from build123d import *

# Parameters (mm, degrees)
CROQUIS1_R                 = 15.5
CROQUIS1_R_2               = 1.5
SALIENTE_EXTRUIR1_DEPTH    = 18.25
CROQUIS2_R                 = 9
CORTAR_EXTRUIR1_DEPTH      = 10
CROQUIS3_R                 = 16.5
CROQUIS3_R_2               = 15.5
SALIENTE_EXTRUIR2_DEPTH    = 1.5
SALIENTE_EXTRUIR3_START    = -1.5
CROQUIS4_R                 = 16.5
CROQUIS4_R_2               = 15.5
SALIENTE_EXTRUIR3_DEPTH    = 1.5
CROQUIS5_W                 = 3
CROQUIS5_H                 = 6.34
CORTAR_EXTRUIR2_DEPTH      = 6.25
CORTAR_EXTRUIR3_DEPTH      = 8
CORTAR_EXTRUIR3_DEPTH_BACK = 9.75
CROQUIS7_R                 = 1.625
CROQUIS8_R                 = 1.625
CORTAR_EXTRUIR4_DEPTH      = 8.25
CORTAR_EXTRUIR7_START      = 15.25
CROQUIS9_R                 = 15.5
CROQUIS9_R_2               = 14.5
CORTAR_EXTRUIR7_DEPTH      = 15.25
CROQUIS11_R                = 16.5
CROQUIS11_R_2              = 9
SALIENTE_EXTRUIR4_DEPTH    = 3.75
CROQUIS12_R                = 16.5
CROQUIS12_R_2              = 14.5
CORTAR_EXTRUIR8_DEPTH      = 3.75


with BuildPart() as part:
    # Croquis1 → Saliente-Extruir1 (new body)
    with BuildSketch(Plane.XY):
        with Locations((-6.34746922, -2.918376653)):
            Circle(CROQUIS1_R)
        with Locations((-6.34746922, -2.918376653)):
            Circle(CROQUIS1_R_2, mode=Mode.SUBTRACT)
    extrude(amount=-SALIENTE_EXTRUIR1_DEPTH)

    # Croquis2 → Cortar-Extruir1 (cut)
    with BuildSketch(Plane(origin=(0, 0, -18.25), x_dir=(-1, 0, 0), z_dir=(0, 0, -1))):
        with Locations((6.34746922, -2.918376653)):
            Circle(CROQUIS2_R)
    extrude(amount=-CORTAR_EXTRUIR1_DEPTH, mode=Mode.SUBTRACT)

    # Croquis3 → Saliente-Extruir2 (add)
    with BuildSketch(Plane.XY):
        with Locations((-6.34746922, -2.918376653)):
            Circle(CROQUIS3_R)
        with Locations((-6.34746922, -2.918376653)):
            Circle(CROQUIS3_R_2, mode=Mode.SUBTRACT)
    extrude(amount=-SALIENTE_EXTRUIR2_DEPTH)

    # Croquis4 → Saliente-Extruir3 (add)
    with BuildSketch(Plane(origin=(0, 0, -18.25), x_dir=(-1, 0, 0), z_dir=(0, 0, -1)).offset(SALIENTE_EXTRUIR3_START)):
        with Locations(Location((6.34746922, -2.918376653, 0), (0, 0, 180))):
            Circle(CROQUIS4_R)
        with Locations(Location((6.34746922, -2.918376653, 0), (0, 0, 180))):
            Circle(CROQUIS4_R_2, mode=Mode.SUBTRACT)
    extrude(amount=SALIENTE_EXTRUIR3_DEPTH)

    # Croquis5 → Cortar-Extruir2 (cut)
    with BuildSketch(Plane.XY):
        with Locations((-0.34746922, -2.918376653)):
            Rectangle(CROQUIS5_W, CROQUIS5_H)
    extrude(amount=-CORTAR_EXTRUIR2_DEPTH, mode=Mode.SUBTRACT)

    # Croquis7 → Cortar-Extruir3 (cut, two sides: drawn at the far end of the back side and taken through both)
    with BuildSketch(Plane.ZY.offset(-1.15253078).offset(-CORTAR_EXTRUIR3_DEPTH_BACK)):
        with Locations((-3.125, -2.918376653)):
            Circle(CROQUIS7_R)
    extrude(amount=CORTAR_EXTRUIR3_DEPTH + CORTAR_EXTRUIR3_DEPTH_BACK, mode=Mode.SUBTRACT)

    # Croquis8 → Cortar-Extruir4 (cut)
    with BuildSketch(Plane.XY):
        with Locations((-6.34746922, -2.918376653)):
            Circle(CROQUIS8_R)
    extrude(amount=-CORTAR_EXTRUIR4_DEPTH, mode=Mode.SUBTRACT)

    # Croquis9 → Cortar-Extruir7 (cut)
    with BuildSketch(Plane.XY.offset(-16.75).offset(CORTAR_EXTRUIR7_START)):
        with Locations((-6.34746922, -2.918376653)):
            Circle(CROQUIS9_R)
        with Locations((-6.34746922, -2.918376653)):
            Circle(CROQUIS9_R_2, mode=Mode.SUBTRACT)
    extrude(amount=-CORTAR_EXTRUIR7_DEPTH, mode=Mode.SUBTRACT)

    # Croquis11 → Saliente-Extruir4 (add)
    with BuildSketch(Plane(origin=(0, 0, -18.25), x_dir=(-1, 0, 0), z_dir=(0, 0, -1))):
        with Locations(Location((6.34746922, -2.918376653, 0), (0, 0, 180))):
            Circle(CROQUIS11_R)
        with Locations((6.34746922, -2.918376653)):
            Circle(CROQUIS11_R_2, mode=Mode.SUBTRACT)
    extrude(amount=SALIENTE_EXTRUIR4_DEPTH)

    # Croquis12 → Cortar-Extruir8 (cut)
    with BuildSketch(Plane.XY.offset(-16.75)):
        with Locations(Location((-6.34746922, -2.918376653, 0), (0, 0, 180))):
            Circle(CROQUIS12_R)
        with Locations((-6.34746922, -2.918376653)):
            Circle(CROQUIS12_R_2, mode=Mode.SUBTRACT)
    extrude(amount=-CORTAR_EXTRUIR8_DEPTH, mode=Mode.SUBTRACT)


solid = part.part
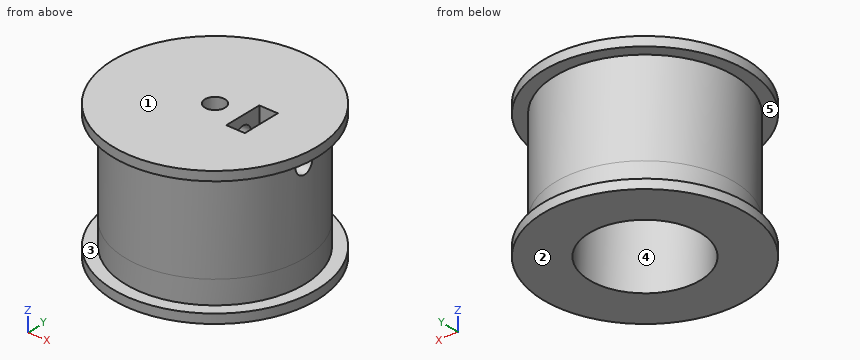
Work out the finished part from the listing and answer in its coordinate system (mm). Face numbers are marked on the shaded views. A direction names the side the tool comes from. Round coordinates to 2 decimals unless told otherwise and drop trailing zeros. Write each loop counter-clockwise with the first axis right and the second up, starting at its lowest first coordinate (ties: lowest second). Pieces come first, ordered by that corner, then holes.
1) Straight lines are drawn through the part: line 1 (Y direction, x = 1, z = -2); line 2 (Z direction, x = -5.5, y = 0.5); line 3 (Y direction, x = -13, z = -8.5). For each, find the intervals that lie inside material, in ascending order.
2) A cutting plane is placed at D-D (x = -20). Give the vertices of the cut face in (y, z).
3) A cutting plane is placed at C-C (z = -5.25). Give the vertices of the cut face in (x, y) (3 decimals), plus the area to 3 significant figures.
4) A tool of negligible diameter and unlimited length cuts with its end or side. For the marked faces 4 and 5, from which of +Z, -Z, +X, -X, +Y, -Y can it reach the whole face along a straight path? Write none if from no direction.
5) The mould has two halves that part along Z. Classify the marked faces 1, 2 and 3: pulls with the +Z half, pulls with the -Z half, needs draft (parallel to the pull), parting line crosses it, or undercut.
6) A cutting plane is placed at A-A (y = -3.5). Give the number of separate pieces and of enclosed holes in the cut face, plus the area to 3 significant figures.
7) Given pin 1 Ø5 at (y, z) = (8, -8) entering from -X; pin 2 Ø10 at (x, z) = (5.5, -10.5) entering from +Y; pin 3 Ø2.5 at (x, y) = (-0.5, -2.5) entering from +Z; pin 4 Ø2.5 at (x, y) = (-6.35, -2.92) entering from +Z, each flat-ended and moving along its own axis, determine where each tip first touches the part or whether it passes through.
Completed:
1. line 1: y = -15.42 to -6.09, 0.25 to 9.58
1. line 2: z = -8.25 to 0
1. line 3: y = -15.8 to -8.98, 3.14 to 9.97
2. outline: (-12.18, -22) - (6.35, -22) - (6.35, -20.5) - (1.97, -20.5) - (1.97, -1.5) - (6.35, -1.5) - (6.35, 0) - (-12.18, 0) - (-12.18, -1.5) - (-7.8, -1.5) - (-7.8, -20.5) - (-12.18, -20.5) - close
3. outline: circle Ø29 at (-6.347, -2.918); hole circle Ø3.25 at (-6.347, -2.918); hole (-1.847, -6.088) - (1.153, -6.088) - (1.153, 0.252) - (-1.847, 0.252) - close
3. area: 633 mm2
4. face 4: -Z
4. face 5: none
5. face 1: pulls with the +Z half
5. face 2: pulls with the -Z half
5. face 3: undercut
6. separate pieces: 4
6. enclosed holes: 0
6. area: 328 mm2
7. pin 1: stops at x = -18.15
7. pin 2: stops at y = 9.86
7. pin 3: stops at z = -6.25
7. pin 4: passes through
